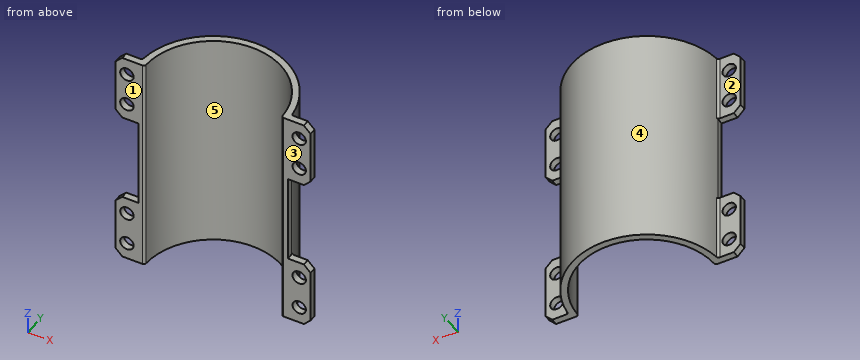
```python
from build123d import *

# Parameters (mm, degrees)
BOSS_EXTRUDE1_DEPTH     = 100
SKETCH3_W               = 10.134598759
SKETCH3_H               = 40
CUT_EXTRUDE1_DEPTH      = 60
SKETCH4_R               = 3
CUT_EXTRUDE2_DEPTH      = 60
MIRROR4_COPY_1_SKETCH_R = 3
MIRROR4_COPY_1_DEPTH    = 60
CHAMFER1_SIZE           = 3
FILLET1_R               = 1


with BuildPart() as part:
    # Sketch1 → Boss-Extrude1 (new body)
    with BuildSketch(Plane.XY):
        with BuildLine():
            Line((-43.5, 0), (-33.5, 0))
            ThreePointArc((-33.5, 0), (-33.466333393, 1.501508976), (-33.365401241, 3))
            Line((-33.365401241, 3), (-43.5, 3))
            Line((-43.5, 3), (-43.5, 0))
        make_face()
        with BuildLine():
            Line((-33.5, 0), (-30.5, 0))
            ThreePointArc((-30.5, 0), (0, 30.5), (30.5, 0))
            Line((30.5, 0), (33.5, 0))
            ThreePointArc((33.5, 0), (33.466333393, 1.501508976), (33.365401241, 3))
            ThreePointArc((33.365401241, 3), (0, 33.5), (-33.365401241, 3))
            ThreePointArc((-33.365401241, 3), (-33.466333393, 1.501508976), (-33.5, 0))
        make_face()
        with BuildLine():
            ThreePointArc((33.365401241, 3), (33.466333393, 1.501508976), (33.5, 0))
            Line((33.5, 0), (43.5, 0))
            Line((43.5, 0), (43.5, 3))
            Line((43.5, 3), (33.365401241, 3))
        make_face()
    extrude(amount=BOSS_EXTRUDE1_DEPTH)

    # Sketch3 → Cut-Extrude1 (cut)
    with BuildSketch(Plane(origin=(0, 3, 0), x_dir=(1, 0, 0), z_dir=(0, 1, 0))):
        with Locations((38.432700621, -50)):
            Rectangle(SKETCH3_W, SKETCH3_H)
        with Locations((-38.432700621, -50)):
            Rectangle(SKETCH3_W, SKETCH3_H)
    extrude(amount=-CUT_EXTRUDE1_DEPTH, mode=Mode.SUBTRACT)

    # Sketch4 → Cut-Extrude2 (cut)
    with BuildSketch(Plane(origin=(0, 3, 0), x_dir=(1, 0, 0), z_dir=(0, 1, 0))):
        with Locations((38.432700621, -22.5)):
            Circle(SKETCH4_R)
        with Locations((38.432700621, -7.5)):
            Circle(SKETCH4_R)
    cut_extrude2 = extrude(amount=-CUT_EXTRUDE2_DEPTH, mode=Mode.SUBTRACT)

    # Mirror3: Cut-Extrude2 across plane
    add(cut_extrude2.mirror(Plane(origin=(0, 0, 50), x_dir=(1, 0, 0), z_dir=(0, 0, -1))), mode=Mode.SUBTRACT)

    # Mirror4: Cut-Extrude2 across plane
    add(cut_extrude2.mirror(Plane(origin=(0, 0, 0), x_dir=(0, 0, 1), z_dir=(1, 0, 0))), mode=Mode.SUBTRACT)

    # Mirror4 copy 1 sketch → Mirror4 copy 1 (cut)
    with BuildSketch(Plane(origin=(0, 3, 100), x_dir=(-1, 0, 0), z_dir=(0, 1, 0))):
        with Locations((38.432700621, -22.5)):
            Circle(MIRROR4_COPY_1_SKETCH_R)
        with Locations((38.432700621, -7.5)):
            Circle(MIRROR4_COPY_1_SKETCH_R)
    extrude(amount=-MIRROR4_COPY_1_DEPTH, mode=Mode.SUBTRACT)

    # Chamfer1
    chamfer1_edges = [part.edges().sort_by_distance(p)[0] for p in [
        (-43.5, 1.5, 0),
        (43.5, 1.5, 0),
        (43.5, 1.5, 100),
        (-43.5, 1.5, 70),
        (-43.5, 1.5, 30),
        (43.5, 1.5, 30),
        (43.5, 1.5, 70),
        (-43.5, 1.5, 100),
    ]]
    chamfer(chamfer1_edges, length=CHAMFER1_SIZE)

    # Fillet1
    fillet1_edges = [part.edges().sort_by_distance(p)[0] for p in [
        (-33.365401241, 3, 85),
        (33.365401241, 3, 85),
        (30.5, 0, 50),
        (-30.5, 0, 50),
        (-33.365401241, 3, 15),
        (33.365401241, 3, 15),
    ]]
    fillet(fillet1_edges, radius=FILLET1_R)


solid = part.part
```
Geometry: final body of the model. Coordinates: model frame, mm. Face numbers are marked on the shaded views. A direction names the side the tool comes from. Coordinates: 2 decimals unless noted, no trailing zeros. Order: outer loops, then holes, each group sorted by start corner. A loop starts at its lowest first (then second) coordinate and runs counter-clockwise, first axis right, second up. Notation, with made-up numbers: M 1,-34 L 38,-34 A11 ccw 38,-15 Z; hole C 34.5,32 d6. An arc over 180 degrees is marked long. Answer in a Markdown table with one row per item. Add a question column.
Q1. Section query C-C on y = 10. Return the cut outline in (x, z), and give its area (3 significant figures).
Q2. Contact query for flat-ended pins moving along their axis: P1, Ø5, axis at y = 11.5, z = 47, coming from the -X side; P2, Ø3, axis at x = 41, z = 89, coming from the +Y side; P3, Ø0.9, axis at y = 1, z = 42.5, coming from the -X side. Output: stop coordinate, or through.
Q3. Section query D-D on y = 18. Return the cut outline in (x, z).
Q4. Mould query, pull axis X, two halves, no side actions, for the marked faces 3, 4 and 5. Classes: released by +X, released by -X, zero draft, split by the parting line, or undercut.
Q5. Line query: L1, parallel to X at y = 1.25, z = 22.5; L2, parallel to X at y = 1.85, z = 22.5; L3, parallel to X at y = 14.5, z = 26.5. Output: solid intervals per line, ascending.
Q6. Section query B-B on x = 37. Return the cut outline in (y, z), and give its area (3 significant figures).
Q7. Reachability of the marked faces 1 and 2 from +Z, -Z, +X, -X, +Y, -Y: full face, straight path, thin tool, end or side. Return the list, or none.
Completed:
| question | item | result |
|---|---|---|
| 1 | outline | M -31.97,0 L -28.81,0 L -28.81,100 L -31.97,100 Z; M 28.81,0 L 31.97,0 L 31.97,100 L 28.81,100 Z |
| 1 | area | 632 mm2 |
| 2 | P1 | stops at x = -32.27 |
| 2 | P2 | stops at y = 3 |
| 2 | P3 | stops at x = -33.37 |
| 3 | outline | M -28.25,0 L -24.62,0 L -24.62,100 L -28.25,100 Z; M 24.62,0 L 28.25,0 L 28.25,100 L 24.62,100 Z |
| 4 | face 3 | zero draft |
| 4 | face 4 | split by the parting line |
| 4 | face 5 | undercut |
| 5 | L1 | x = -43.5 to -41.43, -35.43 to -30.47, 30.47 to 35.43, 41.43 to 43.5 |
| 5 | L2 | x = -43.5 to -41.43, -35.43 to -30.44, 30.44 to 35.43, 41.43 to 43.5 |
| 5 | L3 | x = -30.2 to -26.83, 26.83 to 30.2 |
| 6 | outline | M 0,0 L 3,0 L 3,4.86 L 0,4.86 Z; M 0,10.14 L 3,10.14 L 3,19.86 L 0,19.86 Z; M 0,25.14 L 3,25.14 L 3,30 L 0,30 Z; M 0,70 L 3,70 L 3,74.86 L 0,74.86 Z; M 0,80.14 L 3,80.14 L 3,89.86 L 0,89.86 Z; M 0,95.14 L 3,95.14 L 3,100 L 0,100 Z |
| 6 | area | 117 mm2 |
| 7 | face 1 | +Z, -Z, +X, -X, -Y |
| 7 | face 2 | +Z, -Z, -X, +Y |
